Geometry: final body of the model. Coordinates: model frame, mm. Give positions to 0.01 mm unless a question says otherwise; leave off trailing zeros. Write each loop counter-clockwise with the first axis right and the second up, starting at its lowest first coordinate (ties: lowest second). Pieces come first, ordered by that corner, then holes. Notation, with made-up numbers: (71, -5.75) -> (129, -5.75) arc R15 cw to (129, 14.25) -> close; hole circle Ø11 at (56.25, 58). An arc over 180 degrees is marked (long way). Use CSV: the item, a comma, the result in double quotes. Start each with the question number.
1) Section A-A (x = -2.5). Output: boundary loops of the cut face in (y, z).
2) Section C-C (z = -56.3). Count the separate pieces of the cut face and the enclosed holes in it, plus the area to 3 significant figures.
3) Material intervals for line 1 (X direction, y = 1.5, z = -56.35); line 2 (X direction, y = 8, z = -56.3) (3 decimals), sorted ascending. Write a range as [from, to].
4) Contact query for a flat-ended pin moving along its axis: P1, Ø1.5, axis at x = -6.5, y = 131, coming from the -Z side. Output: stop coordinate, or through.
5) Section B-B (y = 115). Output: boundary loops of the cut face in (x, z), plus the area to 4 significant figures.
```python
from build123d import *

# Parameters (mm, degrees)
PAD024_DEPTH = 0.15
PAD025_DEPTH = 0.15
PAD026_DEPTH = 0.15
PAD027_DEPTH = 0.15
PAD028_DEPTH = 0.15
PAD029_DEPTH = 0.15
BOX011_W     = 32
BOX011_H     = 10
BOX011_DEPTH = 10
PAD030_DEPTH = 0.15
PAD023_DEPTH = 0.15


with BuildPart() as battery_connector008:
    # Sketch038 → Pad024 (new body)
    with BuildSketch(Plane.XY):
        Polygon((-15.25, -15), (-15.25, 7.5), (-12.25, 7.5), (-12.25, 0.25), (-11.25, 0.25), (-11.25, 7.5), (11.25, 7.5), (11.25, 0.25), (12.25, 0.25), (12.25, 7.5), (15.25, 7.5), (15.25, -15), (7.625, -15), (7.625, 0.25), (-7.625, 0.25), (-7.625, -15), align=None)
    extrude(amount=PAD024_DEPTH)


with BuildPart() as battery_connector008_1:
    # Body032 placement: moved
    add(battery_connector008.part.moved(Location((0, 22.5, 0))))


with BuildPart() as battery_connector009:
    # Sketch039 → Pad025 (new body)
    with BuildSketch(Plane.XY):
        Polygon((-15.25, -15), (-15.25, 7.5), (-12.25, 7.5), (-12.25, 0.25), (-11.25, 0.25), (-11.25, 7.5), (11.25, 7.5), (11.25, 0.25), (12.25, 0.25), (12.25, 7.5), (15.25, 7.5), (15.25, -15), (7.625, -15), (7.625, 0.25), (-7.625, 0.25), (-7.625, -15), align=None)
    extrude(amount=PAD025_DEPTH)


with BuildPart() as battery_connector009_1:
    # Body033 placement: moved
    add(battery_connector009.part.moved(Location((0, 45, 0))))


with BuildPart() as battery_connector010:
    # Sketch040 → Pad026 (new body)
    with BuildSketch(Plane.XY):
        Polygon((-15.25, -15), (-15.25, 7.5), (-12.25, 7.5), (-12.25, 0.25), (-11.25, 0.25), (-11.25, 7.5), (11.25, 7.5), (11.25, 0.25), (12.25, 0.25), (12.25, 7.5), (15.25, 7.5), (15.25, -15), (7.625, -15), (7.625, 0.25), (-7.625, 0.25), (-7.625, -15), align=None)
    extrude(amount=PAD026_DEPTH)


with BuildPart() as battery_connector010_1:
    # Body034 placement: moved
    add(battery_connector010.part.moved(Location((0, 67.5, 0))))


with BuildPart() as battery_connector011:
    # Sketch041 → Pad027 (new body)
    with BuildSketch(Plane.XY):
        Polygon((-15.25, -15), (-15.25, 7.5), (-12.25, 7.5), (-12.25, 0.25), (-11.25, 0.25), (-11.25, 7.5), (11.25, 7.5), (11.25, 0.25), (12.25, 0.25), (12.25, 7.5), (15.25, 7.5), (15.25, -15), (7.625, -15), (7.625, 0.25), (-7.625, 0.25), (-7.625, -15), align=None)
    extrude(amount=PAD027_DEPTH)


with BuildPart() as battery_connector011_1:
    # Body035 placement: moved
    add(battery_connector011.part.moved(Location((0, 90, 0))))


with BuildPart() as battery_connector012:
    # Sketch042 → Pad028 (new body)
    with BuildSketch(Plane.XY):
        Polygon((-15.25, -15), (-15.25, 7.5), (-12.25, 7.5), (-12.25, 0.25), (-11.25, 0.25), (-11.25, 7.5), (11.25, 7.5), (11.25, 0.25), (12.25, 0.25), (12.25, 7.5), (15.25, 7.5), (15.25, -15), (7.625, -15), (7.625, 0.25), (-7.625, 0.25), (-7.625, -15), align=None)
    extrude(amount=PAD028_DEPTH)


with BuildPart() as battery_connector012_1:
    # Body036 placement: moved
    add(battery_connector012.part.moved(Location((0, 112.5, 0))))


with BuildPart() as battery_connector013:
    # Sketch043 → Pad029 (new body)
    with BuildSketch(Plane.XY):
        Polygon((-15.25, -15), (-15.25, 7.5), (-12.25, 7.5), (-12.25, 0.25), (-11.25, 0.25), (-11.25, 7.5), (11.25, 7.5), (11.25, 0.25), (12.25, 0.25), (12.25, 7.5), (15.25, 7.5), (15.25, -15), (7.625, -15), (7.625, 0.25), (-7.625, 0.25), (-7.625, -15), align=None)
    extrude(amount=PAD029_DEPTH)


with BuildPart() as battery_connector013_1:
    # Body037 placement: moved
    add(battery_connector013.part.moved(Location((0, 135, 0))))


with BuildPart() as cube011:
    # Box011 → Box011 (new body)
    with BuildSketch(Plane(origin=(-16, 157.75, -5), x_dir=(1, 0, 0), z_dir=(0, 0, 1))):
        with Locations((16, 5)):
            Rectangle(BOX011_W, BOX011_H)
    extrude(amount=BOX011_DEPTH)


with BuildPart() as cut004:
    # Sketch044 → Pad030 (new body)
    with BuildSketch(Plane.XY):
        Polygon((-15.25, -15), (-15.25, 7.5), (-12.25, 7.5), (-12.25, 0.25), (-11.25, 0.25), (-11.25, 7.5), (11.25, 7.5), (11.25, 0.25), (12.25, 0.25), (12.25, 7.5), (15.25, 7.5), (15.25, -15), (7.625, -15), (7.625, 0.25), (-7.625, 0.25), (-7.625, -15), align=None)
    extrude(amount=PAD030_DEPTH)


with BuildPart() as cut004_1:
    # Body038 placement: moved
    add(cut004.part.moved(Location((0, 157.5, 0))))

    # Cut004: cut Cube011
    add(cube011.part, mode=Mode.SUBTRACT)


with BuildPart() as batteryconnector:
    # Sketch037 → Pad023 (new body)
    with BuildSketch(Plane.XY):
        Polygon((-15.25, -15), (-15.25, 7.5), (-12.25, 7.5), (-12.25, 0.25), (-11.25, 0.25), (-11.25, 7.5), (11.25, 7.5), (11.25, 0.25), (12.25, 0.25), (12.25, 7.5), (15.25, 7.5), (15.25, -15), (7.625, -15), (7.625, 0.25), (-7.625, 0.25), (-7.625, -15), align=None)
    extrude(amount=PAD023_DEPTH)

    # Fusion: union Battery Connector008, Battery Connector009, Battery Connector010, Battery Connector011, Battery Connector012, Battery Connector013, Cut004
    add(battery_connector008_1.part)
    add(battery_connector009_1.part)
    add(battery_connector010_1.part)
    add(battery_connector011_1.part)
    add(battery_connector012_1.part)
    add(battery_connector013_1.part)
    add(cut004_1.part)


with BuildPart() as batteryconnector_1:
    # refine placement: moved
    add(batteryconnector.part.moved(Location((0, -1.273, -56.4))))


solid = batteryconnector_1.part
```
Answers follow:
1,outline,"(-1.02, -56.4) -> (6.23, -56.4) -> (6.23, -56.25) -> (-1.02, -56.25) -> close; (21.48, -56.4) -> (28.73, -56.4) -> (28.73, -56.25) -> (21.48, -56.25) -> close; (43.98, -56.4) -> (51.23, -56.4) -> (51.23, -56.25) -> (43.98, -56.25) -> close; (66.48, -56.4) -> (73.73, -56.4) -> (73.73, -56.25) -> (66.48, -56.25) -> close; (88.98, -56.4) -> (96.23, -56.4) -> (96.23, -56.25) -> (88.98, -56.25) -> close; (111.48, -56.4) -> (118.73, -56.4) -> (118.73, -56.25) -> (111.48, -56.25) -> close; (133.98, -56.4) -> (141.23, -56.4) -> (141.23, -56.25) -> (133.98, -56.25) -> close"
2,separate pieces,"1"
2,enclosed holes,"20"
2,area,"3,310 mm^2"
3,line 1,"x = [-15.25, -12.25], [-11.25, 11.25], [12.25, 15.25]"
3,line 2,"x = [-15.25, -7.625], [7.625, 15.25]"
4,P1,"passes through"
5,outline,"(-15.25, -56.4) -> (-12.25, -56.4) -> (-12.25, -56.25) -> (-15.25, -56.25) -> close; (-11.25, -56.4) -> (11.25, -56.4) -> (11.25, -56.25) -> (-11.25, -56.25) -> close; (12.25, -56.4) -> (15.25, -56.4) -> (15.25, -56.25) -> (12.25, -56.25) -> close"
5,area,"4.275 mm^2"
